Verification items for this drawing (mm, ordinates from the low corner). Give positions to 0.01 mm unless a question says otherwise; leave off trailing zeros. Order: outer loops, then holes, each group sorted by start corner. A loop starts at its lowest first (then second) coordinate and runs counter-clockwise, first axis right, second up. Notation, with made-up numbers: (56, 19.5) - (64, 19.5) arc R13 ccw to (64, 26.5) - close; hole circle Ø10 at (53.25, 50). An arc over 180 degrees is marked (long way). Put each result on its own line as item: value. Start each with the question number.
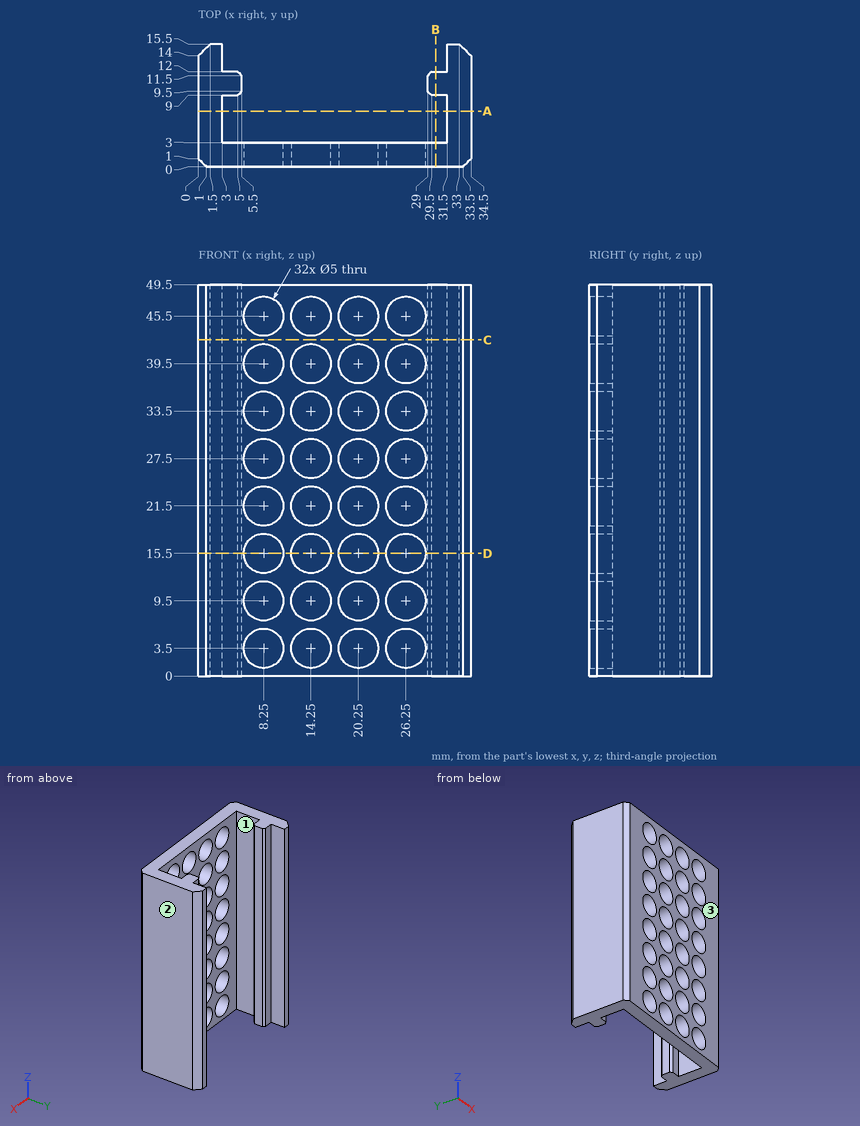
Item 1: Cross-section at D-D (z = 15.5). Count the separate pieces of the cut face and the enclosed holes in it, and give its area (3 significant figures).
Item 2: Cross-section at B-B (x = 30). Enter the section's corners in (y, z), and give its area (3 significant figures).
Item 3: Cross-section at A-A (y = 7). Enter the section's corners in (x, z).
Item 4: Release check for a two-part mould opening along Y. For the marked faces 1, 2 and 3 record: +Y half, -Y half, draft (parallel to the pull), parting line (faces both ways), or undercut.
Item 5: Cross-section at C-C (z = 42.5). Enter the section's corners in (x, y).
Item 6: Gauge pin test, flat ends, axial feed: pin 1 Ø1.5 at (x, y) = (27.5, 8.5) entering from -Z; pin 2 Ø8 at (x, z) = (20.25, 27.5) entering from +Y; pin 3 Ø8 at (x, z) = (26.25, 21.5) entering from +Y. Record the tip position at first contact, or that the pin passes through.
Item 7: Thickness scan on line 1 along Y through (x, z) = (30, 5); line 2 along X through (y, z) = (10.75, 46); line 3 along X through (y, z) = (6.5, 21.5). Record the ranges inside material, lowest first.
Recorded:
1. separate pieces: 5
1. enclosed holes: 0
1. area: 130 mm^2
2. outline: (0, 0) - (3, 0) - (3, 49.5) - (0, 49.5) - close; (9, 0) - (12, 0) - (12, 49.5) - (9, 49.5) - close
2. area: 297 mm^2
3. outline: (0, 0) - (3, 0) - (3, 49.5) - (0, 49.5) - close; (31.5, 0) - (34.5, 0) - (34.5, 49.5) - (31.5, 49.5) - close
4. face 1: undercut
4. face 2: draft
4. face 3: -Y half
5. outline: (0, 1) - (1, 0) - (33.5, 0) - (34.5, 1) - (34.5, 14) - (33, 15.5) - (31.5, 15.5) - (31.5, 12) - (29.5, 12) - (29, 11.5) - (29, 9.5) - (29.5, 9) - (31.5, 9) - (31.5, 3) - (3, 3) - (3, 9) - (5, 9) - (5.5, 9.5) - (5.5, 11.5) - (5, 12) - (3, 12) - (3, 15.5) - (1.5, 15.5) - (0, 14) - close
6. pin 1: passes through
6. pin 2: stops at y = 3
6. pin 3: stops at y = 12
7. line 1: y = 0 to 3, 9 to 12
7. line 2: x = 0 to 5.5, 29 to 34.5
7. line 3: x = 0 to 3, 31.5 to 34.5
